Read the model definition and answer for the solid it produces. Units are mm, in the model's axes. Face numbers are marked on the shaded views. A direction names the side the tool comes from. Coordinates: 2 decimals unless noted, no trailing zeros. Loops run counter-clockwise (first coordinate to the right, second up) from the corner with the lowest first, then second, coordinate; pieces in that order, holes last. Notation, with made-up numbers: (49, 16.5) -> (69, 16.5) arc R20 cw to (69, 32.5) -> close; hole circle Ø6 at (40.25, 19.5). An arc over 180 degrees is marked (long way). Answer as a JSON object with one key per item and string values. Group by question number.
Q1. Each of these flat-tipped pins is pushed along its axis until it touches: P1, Ø4, axis at x = -28.5, z = 49, coming from the -Y side; P2, Ø1.5, axis at x = 40, z = 2, coming from the -Y side; P3, Ø7, axis at x = -27.5, y = 86, coming from the +Z side; P4, Ø12, axis at y = 10.5, z = 27.5, coming from the +X side. Where does it stop, or does it pass through?
Q2. Determine the mould class of the marked faces 1, 2, 3 and 4 for opening direction Z: released by +Z, released by -Z, zero draft, split by the parting line, or undercut.
Q3. The part is cut by section B-B on x = 56.5. Write down the section's boundary in (y, z) (3 decimals).
Q4. The part is cut by section A-A on z = 6. Write down the section's boundary in (x, y) (3 decimals), and give its area (3 significant figures).
Q5. The part is cut by section C-C on x = 0. Write down the section's boundary in (y, z) (3 decimals).
Q6. The part is cut by section D-D on z = 50. State how many separate pieces and enclosed holes the cut face has, and give its area (3 significant figures).
Q7. Straight lines are drawn through the part: line 1 along X through (y, z) = (87.25, 38.1); line 2 along Y through (x, z) = (-44, 24); line 3 along Z through (x, y) = (28.5, 60). For each, find the intervals that lie inside material, in ascending order. Write a range as [from, to].
Q8. For the marked faces 5, 6, 7 and 8, determine the directions among +Z, -Z, +X, -X, +Y, -Y from which every point of the face is accessible in a straight line to the end or side of a thin tool.
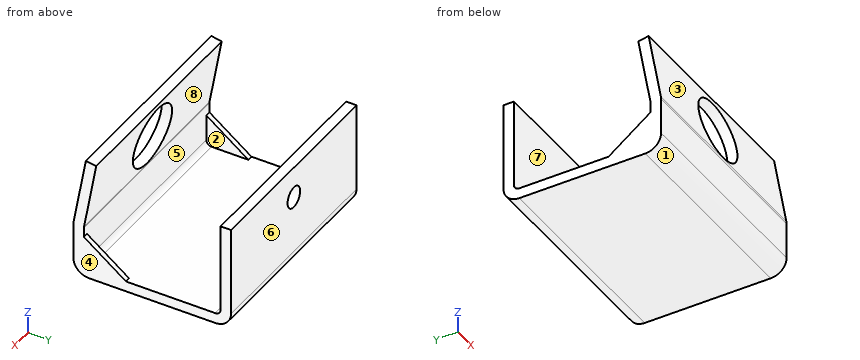
from build123d import *

# Parameters (mm, degrees)
BASE_EXTRUDE_THIN_DEPTH = 63.5
CUT_EXTRUDE1_REACH      = 135.471
SKETCH2_R               = 6.35
BOSS_EXTRUDE1_DEPTH     = 3.175
D_GAGEMENT_00001_D      = 25.4
D_GAGEMENT_00001_DEPTH  = 6.35
D_GAGEMENT_00001_TIP    = 7.630929862
ESQUISSE3_R             = 19.05
ENL_V_MAT_EXTRU_1_DEPTH = 132.649844576


with BuildPart() as part:
    # Sketch1 → Base-Extrude-Thin (new, symmetric)
    with BuildSketch(Plane(origin=(0, 0, 0), x_dir=(0, 0, -1), z_dir=(1, 0, 0))):
        with BuildLine():
            Line((-67.523772904, 7.427557692), (-25.673556457, 0.048235384))
            ThreePointArc((-25.673556457, 0.048235384), (-25.398942977, 0.012081834), (-25.122223493, 0))
            Line((-25.122223493, 0), (-3.175, 0))
            ThreePointArc((-3.175, 0), (-0.92993597, 0.92993597), (0, 3.175))
            Line((0, 3.175), (0, 79.375))
            ThreePointArc((0, 79.375), (-0.92993597, 81.62006403), (-3.175, 82.55))
            Line((-3.175, 82.55), (-57.15, 82.55))
            Line((-57.15, 82.55), (-57.15, 88.9))
            Line((-57.15, 88.9), (-3.175, 88.9))
            ThreePointArc((-3.175, 88.9), (3.560192091, 86.110192091), (6.35, 79.375))
            Line((6.35, 79.375), (6.35, 3.175))
            ThreePointArc((6.35, 3.175), (3.560192091, -3.560192091), (-3.175, -6.35))
            Line((-3.175, -6.35), (-25.122223493, -6.35))
            ThreePointArc((-25.122223493, -6.35), (-25.952381943, -6.313754499), (-26.776222386, -6.205293847))
            Line((-26.776222386, -6.205293847), (-68.626438832, 1.174028461))
            Line((-68.626438832, 1.174028461), (-67.523772904, 7.427557692))
        make_face()
    extrude(amount=BASE_EXTRUDE_THIN_DEPTH, both=True)

    # Sketch2 → Cut-Extrude1 (cut, up to next)
    with BuildSketch(Plane(origin=(0, 88.9, 0), x_dir=(-1, 0, 0), z_dir=(0, 1, 0)), mode=Mode.PRIVATE) as cut_extrude1_sk1:
        with Locations(Location((0, 38.1, 0), (0, 0, 90))):
            Circle(SKETCH2_R)
    cut_extrude1_tool1 = extrude(cut_extrude1_sk1.sketch, amount=-CUT_EXTRUDE1_REACH, mode=Mode.PRIVATE) & part.part
    add(cut_extrude1_tool1.solids().sort_by_distance((0, 88.9, 38.1))[0], mode=Mode.SUBTRACT)

    # Sketch3 → Boss-Extrude1 (add)
    with BuildSketch(Plane(origin=(63.5, 0, 0), x_dir=(0, 0, -1), z_dir=(1, 0, 0))):
        with BuildLine():
            Line((-19.05, 0), (-3.175, 0))
            ThreePointArc((-3.175, 0), (-0.92993597, 0.92993597), (0, 3.175))
            Line((0, 3.175), (0, 25.4))
            Line((0, 25.4), (-19.05, 0))
        make_face()
    boss_extrude1 = extrude(amount=-BOSS_EXTRUDE1_DEPTH)

    # Mirror1: Boss-Extrude1 across plane
    add(boss_extrude1.mirror(Plane(origin=(0, 0, 0), x_dir=(0, 0, 1), z_dir=(1, 0, 0))))

    # Dégagement #00001
    with Locations(Plane(origin=(0, -4.34365582, 0.765903716), x_dir=(-1, 0, 0), z_dir=(0, 0.9848077530122081, -0.17364817766693075))):
        with Locations((-4.206462063, 49.405030417)):
            Hole(D_GAGEMENT_00001_D / 2, depth=D_GAGEMENT_00001_DEPTH)
            with Locations((0, 0, -(D_GAGEMENT_00001_DEPTH + D_GAGEMENT_00001_TIP / 2))):  # 118° drill point
                Cone(0, D_GAGEMENT_00001_D / 2, D_GAGEMENT_00001_TIP, mode=Mode.SUBTRACT)

    # Esquisse3 → Enlèv. mat.-Extru.1 (cut, through all)
    with BuildSketch(Plane(origin=(0, -4.34365582, 0.765903716), x_dir=(1, 0, 0), z_dir=(0, 0.9848077530122081, -0.1736481776669307))):
        with Locations(Location((0, -45.239836887, 0), (0, 0, 270))):
            Circle(ESQUISSE3_R)
    extrude(amount=-ENL_V_MAT_EXTRU_1_DEPTH, mode=Mode.SUBTRACT)


solid = part.part
Final values:
{
 "1": {"P1": "stops at y = -2.64", "P2": "stops at y = -6.34", "P3": "stops at z = 57.15", "P4": "passes through"},
 "2": {"face 1": "released by -Z", "face 2": "undercut", "face 3": "released by +Z", "face 4": "zero draft"},
 "3": {"outline": "(-6.35, 3.175) arc R9.525 ccw to (3.175, -6.35) -> (79.375, -6.35) arc R9.525 ccw to (88.9, 3.175) -> (88.9, 57.15) -> (82.55, 57.15) -> (82.55, 3.175) arc R3.175 cw to (79.375, 0) -> (3.175, 0) arc R3.175 cw to (0, 3.175) -> (0, 25.122) arc R3.175 cw to (0.048, 25.674) -> (7.428, 67.524) -> (1.174, 68.626) -> (-6.205, 26.776) arc R9.525 ccw to (-6.35, 25.122) -> close"},
 "4": {"outline": "(-63.5, -6.35) -> (63.5, -6.35) -> (63.5, 17.4) -> (60.325, 17.4) -> (60.325, 0) -> (-60.325, 0) -> (-60.325, 17.4) -> (-63.5, 17.4) -> close; (-63.5, 82.55) -> (63.5, 82.55) -> (63.5, 88.9) -> (-63.5, 88.9) -> close", "area": "1,720 mm2"},
 "5": {"outline": "(-6.35, 3.175) arc R9.525 ccw to (3.175, -6.35) -> (79.375, -6.35) arc R9.525 ccw to (88.9, 3.175) -> (88.9, 31.75) -> (82.55, 31.75) -> (82.55, 3.175) arc R3.175 cw to (79.375, 0) -> (3.175, 0) arc R3.175 cw to (0, 3.175) -> (0, 25.122) arc R3.175 cw to (0.048, 25.674) -> (0.204, 26.558) -> (-6.049, 27.661) -> (-6.205, 26.776) arc R9.525 ccw to (-6.35, 25.122) -> close; (0.567, 65.182) -> (6.82, 64.079) -> (7.428, 67.524) -> (1.174, 68.626) -> close; (82.55, 44.45) -> (88.9, 44.45) -> (88.9, 57.15) -> (82.55, 57.15) -> close"},
 "6": {"separate pieces": "3", "enclosed holes": "0", "area": "1,390 mm2"},
 "7": {"line 1": "x = [-63.5, -6.35], [6.35, 63.5]", "line 2": "y = [-6.35, 0], [82.55, 88.9]", "line 3": "z = [-6.35, 0]"},
 "8": {"face 5": "none", "face 6": "+Z, -Z, +X, -X, +Y", "face 7": "+Z, +X, -X", "face 8": "+X, -X"}
}
